from build123d import *

# Parameters (mm, degrees)
BOSS_EXTRUDE1_DEPTH = 3
SKETCH2_R           = 2.125
CUT_EXTRUDE1_DEPTH  = 503.104570782
SKETCH3_R           = 2
CUT_EXTRUDE2_DEPTH  = 503.104570782
SKETCH5_R           = 2.125
CUT_EXTRUDE4_DEPTH  = 10
FILLET1_R           = 20
SKETCH6_R           = 2.125
CUT_EXTRUDE5_DEPTH  = 503.104570782
SKETCH8_R           = 2.1
CUT_EXTRUDE6_DEPTH  = 10
SKETCH7_R           = 2.1
CUT_EXTRUDE7_DEPTH  = 10


with BuildPart() as part:
    # Sketch1 → Boss-Extrude1 (new body)
    with BuildSketch(Plane(origin=(0, 0, 0), x_dir=(1, 0, 0), z_dir=(0, 1, 0))):
        Polygon((-110, 350), (-110, 108), (-338, 108), (-338, 130), (-360, 130), (-360, -130), (-338, -130), (-338, -108), (-110, -108), (-110, -350), (110, -350), (110, -108), (338, -108), (338, -130), (360, -130), (360, 130), (338, 130), (338, 108), (110, 108), (110, 350), align=None)
    extrude(amount=BOSS_EXTRUDE1_DEPTH)

    # Sketch2 → Cut-Extrude1 (cut, through all)
    with BuildSketch(Plane(origin=(0, 3, 0), x_dir=(1, 0, 0), z_dir=(0, 1, 0))):
        with Locations(Location((310, 47.5, 0), (0, 0, 270))):
            Circle(SKETCH2_R)
        with Locations(Location((285, 47.5, 0), (0, 0, 270))):
            Circle(SKETCH2_R)
        with Locations(Location((307.5, 17.5, 0), (0, 0, 270))):
            Circle(SKETCH2_R)
        with Locations(Location((307.5, -17.5, 0), (0, 0, 270))):
            Circle(SKETCH2_R)
        with Locations(Location((310, -47.5, 0), (0, 0, 270))):
            Circle(SKETCH2_R)
        with Locations(Location((285, -47.5, 0), (0, 0, 270))):
            Circle(SKETCH2_R)
        with Locations(Location((-285, -47.5, 0), (0, 0, 90))):
            Circle(SKETCH2_R)
        with Locations(Location((-310, -47.5, 0), (0, 0, 90))):
            Circle(SKETCH2_R)
        with Locations(Location((-307.5, -17.5, 0), (0, 0, 90))):
            Circle(SKETCH2_R)
        with Locations(Location((-307.5, 17.5, 0), (0, 0, 90))):
            Circle(SKETCH2_R)
        with Locations(Location((-285, 47.5, 0), (0, 0, 90))):
            Circle(SKETCH2_R)
        with Locations(Location((-310, 47.5, 0), (0, 0, 90))):
            Circle(SKETCH2_R)
        with Locations(Location((47.5, 300, 0), (0, 0, 270))):
            Circle(SKETCH2_R)
        with Locations(Location((47.5, 275, 0), (0, 0, 270))):
            Circle(SKETCH2_R)
        with Locations(Location((-47.5, 275, 0), (0, 0, 90))):
            Circle(SKETCH2_R)
        with Locations(Location((-47.5, 300, 0), (0, 0, 90))):
            Circle(SKETCH2_R)
        with Locations(Location((-47.5, -300, 0), (0, 0, 270))):
            Circle(SKETCH2_R)
        with Locations(Location((-47.5, -275, 0), (0, 0, 270))):
            Circle(SKETCH2_R)
        with Locations(Location((47.5, -275, 0), (0, 0, 90))):
            Circle(SKETCH2_R)
        with Locations(Location((47.5, -300, 0), (0, 0, 90))):
            Circle(SKETCH2_R)
    extrude(amount=-CUT_EXTRUDE1_DEPTH, mode=Mode.SUBTRACT)

    # Sketch3 → Cut-Extrude2 (cut, through all)
    with BuildSketch(Plane(origin=(0, 3, 0), x_dir=(1, 0, 0), z_dir=(0, 1, 0))):
        with Locations(Location((340, 38, 0), (0, 0, 270))):
            Circle(SKETCH3_R)
        with Locations(Location((340, -38, 0), (0, 0, 90))):
            Circle(SKETCH3_R)
        with Locations(Location((-340, -38, 0), (0, 0, 270))):
            Circle(SKETCH3_R)
        with Locations(Location((-340, 38, 0), (0, 0, 90))):
            Circle(SKETCH3_R)
        with Locations(Location((-30, 330, 0), (0, 0, 270))):
            Circle(SKETCH3_R)
        with Locations(Location((30, 330, 0), (0, 0, 90))):
            Circle(SKETCH3_R)
        with Locations(Location((30, -330, 0), (0, 0, 270))):
            Circle(SKETCH3_R)
        with Locations(Location((-30, -330, 0), (0, 0, 90))):
            Circle(SKETCH3_R)
    extrude(amount=-CUT_EXTRUDE2_DEPTH, mode=Mode.SUBTRACT)

    # Sketch5 → Cut-Extrude4 (cut)
    with BuildSketch(Plane(origin=(0, 3, 0), x_dir=(1, 0, 0), z_dir=(0, 1, 0))):
        with Locations(Location((80, 300, 0), (0, 0, 270))):
            Circle(SKETCH5_R)
        with Locations(Location((80, 148.73, 0), (0, 0, 270))):
            Circle(SKETCH5_R)
        with Locations(Location((85.11, 239.365, 0), (0, 0, 270))):
            Circle(SKETCH5_R)
        with Locations(Location((85.11, 209.365, 0), (0, 0, 270))):
            Circle(SKETCH5_R)
        with Locations(Location((100, 148.73, 0), (0, 0, 90))):
            Circle(SKETCH5_R)
        with Locations(Location((100, 300, 0), (0, 0, 90))):
            Circle(SKETCH5_R)
        with Locations(Location((-100, 300, 0), (0, 0, 270))):
            Circle(SKETCH5_R)
        with Locations(Location((-100, 148.73, 0), (0, 0, 270))):
            Circle(SKETCH5_R)
        with Locations(Location((-85.11, 209.365, 0), (0, 0, 90))):
            Circle(SKETCH5_R)
        with Locations(Location((-85.11, 239.365, 0), (0, 0, 90))):
            Circle(SKETCH5_R)
        with Locations(Location((-80, 148.73, 0), (0, 0, 90))):
            Circle(SKETCH5_R)
        with Locations(Location((-80, 300, 0), (0, 0, 90))):
            Circle(SKETCH5_R)
        with Locations(Location((-80, -300, 0), (0, 0, 270))):
            Circle(SKETCH5_R)
        with Locations(Location((-80, -148.73, 0), (0, 0, 270))):
            Circle(SKETCH5_R)
        with Locations(Location((-85.11, -239.365, 0), (0, 0, 270))):
            Circle(SKETCH5_R)
        with Locations(Location((-85.11, -209.365, 0), (0, 0, 270))):
            Circle(SKETCH5_R)
        with Locations(Location((-100, -148.73, 0), (0, 0, 90))):
            Circle(SKETCH5_R)
        with Locations(Location((-100, -300, 0), (0, 0, 90))):
            Circle(SKETCH5_R)
        with Locations(Location((100, -300, 0), (0, 0, 270))):
            Circle(SKETCH5_R)
        with Locations(Location((100, -148.73, 0), (0, 0, 270))):
            Circle(SKETCH5_R)
        with Locations(Location((85.11, -209.365, 0), (0, 0, 90))):
            Circle(SKETCH5_R)
        with Locations(Location((85.11, -239.365, 0), (0, 0, 90))):
            Circle(SKETCH5_R)
        with Locations(Location((80, -148.73, 0), (0, 0, 90))):
            Circle(SKETCH5_R)
        with Locations(Location((80, -300, 0), (0, 0, 90))):
            Circle(SKETCH5_R)
    extrude(amount=-CUT_EXTRUDE4_DEPTH, mode=Mode.SUBTRACT)

    # Fillet1
    fillet1_edges = [part.edges().sort_by_distance(p)[0] for p in [
        (110, 1.5, -108),
        (110, 1.5, 108),
        (-110, 1.5, 108),
        (-110, 1.5, -108),
    ]]
    fillet(fillet1_edges, radius=FILLET1_R)

    # Sketch6 → Cut-Extrude5 (cut, through all)
    with BuildSketch(Plane(origin=(0, 3, 0), x_dir=(1, 0, 0), z_dir=(0, 1, 0))):
        with Locations(Location((53.325901808, -194.747258045, 0), (0, 0, 270))):
            Circle(SKETCH6_R)
        with Locations(Location((-192.747258045, 51.325901808, 0), (0, 0, 270))):
            Circle(SKETCH6_R)
        with Locations(Location((-28.69848481, -112.722871427, 0), (0, 0, 270))):
            Circle(SKETCH6_R)
        with Locations(Location((-110.722871427, -30.69848481, 0), (0, 0, 270))):
            Circle(SKETCH6_R)
        with Locations(Location((64.639610307, -183.433549546, 0), (0, 0, 90))):
            Circle(SKETCH6_R)
        with Locations(Location((-17.384776311, -101.409162928, 0), (0, 0, 90))):
            Circle(SKETCH6_R)
        with Locations(Location((-99.409162928, -19.384776311, 0), (0, 0, 90))):
            Circle(SKETCH6_R)
        with Locations(Location((-181.433549546, 62.639610307, 0), (0, 0, 90))):
            Circle(SKETCH6_R)
        with Locations(Location((-62.639610307, 181.433549546, 0), (0, 0, 270))):
            Circle(SKETCH6_R)
        with Locations(Location((19.384776311, 99.409162928, 0), (0, 0, 270))):
            Circle(SKETCH6_R)
        with Locations(Location((101.409162928, 17.384776311, 0), (0, 0, 270))):
            Circle(SKETCH6_R)
        with Locations(Location((183.433549546, -64.639610307, 0), (0, 0, 270))):
            Circle(SKETCH6_R)
        with Locations(Location((30.69848481, 110.722871427, 0), (0, 0, 90))):
            Circle(SKETCH6_R)
        with Locations(Location((112.722871427, 28.69848481, 0), (0, 0, 90))):
            Circle(SKETCH6_R)
        with Locations(Location((-51.325901808, 192.747258045, 0), (0, 0, 90))):
            Circle(SKETCH6_R)
        with Locations(Location((194.747258045, -53.325901808, 0), (0, 0, 90))):
            Circle(SKETCH6_R)
    extrude(amount=-CUT_EXTRUDE5_DEPTH, mode=Mode.SUBTRACT)

    # Sketch8 → Cut-Extrude6 (cut)
    with BuildSketch(Plane(origin=(0, 3, 0), x_dir=(1, 0, 0), z_dir=(0, 1, 0))):
        with Locations(Location((-40, 35, 0), (0, 0, 270))):
            Circle(SKETCH8_R)
        with Locations(Location((40, 35, 0), (0, 0, 90))):
            Circle(SKETCH8_R)
        with Locations(Location((40, -35, 0), (0, 0, 270))):
            Circle(SKETCH8_R)
        with Locations(Location((-40, -35, 0), (0, 0, 90))):
            Circle(SKETCH8_R)
    extrude(amount=-CUT_EXTRUDE6_DEPTH, mode=Mode.SUBTRACT)

    # Sketch7 → Cut-Extrude7 (cut)
    with BuildSketch(Plane(origin=(0, 3, 0), x_dir=(1, 0, 0), z_dir=(0, 1, 0))):
        with Locations(Location((340, 88, 0), (0, 0, 270))):
            Circle(SKETCH7_R)
        with Locations(Location((340, -88, 0), (0, 0, 90))):
            Circle(SKETCH7_R)
        with Locations(Location((-340, -88, 0), (0, 0, 270))):
            Circle(SKETCH7_R)
        with Locations(Location((-340, 88, 0), (0, 0, 90))):
            Circle(SKETCH7_R)
        with Locations(Location((-90, 330, 0), (0, 0, 270))):
            Circle(SKETCH7_R)
        with Locations(Location((90, 330, 0), (0, 0, 90))):
            Circle(SKETCH7_R)
        with Locations(Location((90, -330, 0), (0, 0, 270))):
            Circle(SKETCH7_R)
        with Locations(Location((-90, -330, 0), (0, 0, 90))):
            Circle(SKETCH7_R)
    extrude(amount=-CUT_EXTRUDE7_DEPTH, mode=Mode.SUBTRACT)


solid = part.part
Geometry check sheet. Reference: the model listing, model coordinates, mm. A direction names the side the tool comes from. Round coordinates to 2 decimals unless told otherwise and drop trailing zeros. Loops run counter-clockwise (first coordinate to the right, second up) from the corner with the lowest first, then second, coordinate; pieces in that order, holes last. Notation, with made-up numbers: (-25.75, 70.5) - (28.25, 70.5) arc R12 ccw to (28.25, 85.5) - close; hole circle Ø8 at (85, 58). An arc over 180 degrees is marked (long way). One line per question, with ' | ' between items. Start each with the question number.
1. Cross-section at B-B on z = -253. Record the cut outline in (x, y), then the cut area to 3 significant figures.
2. Scan lines: line 1 (X direction, y = 2.05, z = -275) (3 decimals); line 2 (Z direction, x = -307.5, y = 1.3) (3 decimals); line 3 (X direction, y = 2.5, z = 125). Record each from-to range of solid material in increasing order. Write a range as [from, to].
3. Cross-section at C-C on y = 1.55. State how many separate pieces and enclosed holes the cut face has, then the cut area to 3 significant figures.
4. Cross-section at A-A on x = -159.5. Record the cut outline in (y, z).
5. Draft check along X on faces 1 (the face through (115.703, 1.521, -114.014)), 2 (the face through (-5, 3, -5)). Enter one of: released by +X, released by -X, zero draft, split by the parting line, or undercut.
6. Tool access check on faces 3 (the face through (116.014, 1.521, 113.703)), 4 (the face through (-115.703, 1.521, -114.014)), 5 (the face through (-5, 0, -5)). Record the directions out of +Z, -Z, +X, -X, +Y, -Y that give a thin tool (end or side, any length) a straight path to the whole face; none if there is none.
7. Depth check by flat-ended pin: pin 1 (1.5 mm diameter, centred on x = 204.5, y = 1, fed in from +Z). Enter the tip coordinate at first touch or a pass-through.
Taken from the geometry:
1) outline: (-110, 0) - (110, 0) - (110, 3) - (-110, 3) - close | area: 660 mm²
2) line 1: [-110, -49.625], [-45.375, 45.375], [49.625, 110] | line 2: [-108, -19.625], [-15.375, 15.375], [19.625, 108] | line 3: [-360, -338], [-110.23, 110.23], [338, 360]
3) separate pieces: 1 | enclosed holes: 80 | area: 263,000 mm²
4) outline: (0, -108) - (3, -108) - (3, 108) - (0, 108) - close
5) face 1: undercut | face 2: zero draft
6) face 3: +Z, +Y, -Y | face 4: -Z, +Y, -Y | face 5: +Z, -Z, +X, -X, -Y
7) pin 1: z = 108
